from build123d import *

# Parameters (mm, degrees)
BOSS_EXTRUDE1_DEPTH   = 38.1
BOSS_EXTRUDE1_2_DEPTH = 38.1
SKETCH2_W             = 7.62
SKETCH2_H             = 5.08
BOSS_EXTRUDE2_DEPTH   = 7.62
SKETCH3_R             = 1.8415
CUT_EXTRUDE1_DEPTH    = 60.428216724
FILLET1_R             = 2.54
FILLET2_R             = 2.54
SKETCH5_W             = 18.161
SKETCH5_H             = 5.08
SKETCH5_W_2           = 21.209
BOSS_EXTRUDE3_DEPTH   = 5.08
SKETCH6_W             = 8.89
SKETCH6_H             = 27.94
CUT_EXTRUDE2_DEPTH    = 63.393930338
SKETCH8_W             = 8.763
SKETCH8_H             = 3.302
BOSS_EXTRUDE4_DEPTH   = 13.97
SKETCH11_R            = 1.8415
CUT_EXTRUDE4_DEPTH    = 62.324385256
CUT_EXTRUDE5_START    = -5.08
SKETCH15_W            = 35.43046
SKETCH15_H            = 22.86
CUT_EXTRUDE5_DEPTH    = 5.08
SKETCH16_R            = 1.8415
BOSS_EXTRUDE5_DEPTH   = 5.08
SKETCH17_W            = 5.08
SKETCH17_H            = 21.717
CUT_EXTRUDE6_DEPTH    = 10.16
CHAMFER1_SIZE         = 2.54


with BuildPart() as part:
    # Sketch1 → Boss-Extrude1 (new body)
    with BuildSketch(Plane(origin=(0, 0, 0), x_dir=(1, 0, 0), z_dir=(0, 1, 0))):
        Polygon((0, 0), (0, 13.71346), (5.08, 13.71346), (5.08, 5.588), (19.05, 5.588), (19.05, 0), align=None)
    extrude(amount=BOSS_EXTRUDE1_DEPTH)

    # Sketch2 → Boss-Extrude2 (add)
    with BuildSketch(Plane.ZY):
        with Locations((-6.85546, 35.56)):
            Rectangle(SKETCH2_W, SKETCH2_H)
        with Locations((-38.73246, 35.56)):
            Rectangle(SKETCH2_W, SKETCH2_H)
    extrude(amount=BOSS_EXTRUDE2_DEPTH)


with BuildPart() as body_2:
    # Sketch1 → Boss-Extrude1 2 (new body)
    with BuildSketch(Plane(origin=(0, 0, 0), x_dir=(1, 0, 0), z_dir=(0, 1, 0))):
        Polygon((0, 31.87446), (5.08, 31.87446), (5.08, 40.00246), (19.05, 40.00246), (19.05, 45.59046), (0, 45.59046), align=None)
    extrude(amount=BOSS_EXTRUDE1_2_DEPTH)



with BuildPart() as boss_extrude2_piece_1:
    # of the separate pieces the step leaves, piece 1, a body of its own (boss_extrude2_pieces)
    add(part.part.solids().sort_by_distance((0, 0, 0))[0])


with BuildPart() as boss_extrude2_piece_2:
    # of the separate pieces the step leaves, piece 2, a body of its own (boss_extrude2_pieces)
    add(part.part.solids().sort_by_distance((0, 38.1, -34.92246))[0])


with BuildPart() as cut_extrude1_tool:
    # Sketch3 → Cut-Extrude1 (new, through all)
    with BuildSketch(Plane(origin=(0, 33.02, 0), x_dir=(-1, 0, 0), z_dir=(0, -1, 0))):
        with Locations(Location((3.996511692, 6.85546, 0), (0, 0, 90))):
            Circle(SKETCH3_R)
        with Locations(Location((3.996511692, 38.73246, 0), (0, 0, 90))):
            Circle(SKETCH3_R)
    extrude(amount=-CUT_EXTRUDE1_DEPTH)


with BuildPart() as boss_extrude2_piece_1_1:
    add(boss_extrude2_piece_1.part)

    # Cut-Extrude1: cut by cut_extrude1_tool
    add(cut_extrude1_tool.part, mode=Mode.SUBTRACT)

    # Fillet1
    fillet1_edges = [boss_extrude2_piece_1_1.edges().sort_by_distance(p)[0] for p in [
        (-7.62, 35.56, -10.66546),
        (-7.62, 35.56, -3.04546),
    ]]
    fillet(fillet1_edges, radius=FILLET1_R)


with BuildPart() as boss_extrude2_piece_2_1:
    add(boss_extrude2_piece_2.part)

    # Cut-Extrude1: cut by cut_extrude1_tool
    add(cut_extrude1_tool.part, mode=Mode.SUBTRACT)

    # Fillet2
    fillet2_edges = [boss_extrude2_piece_2_1.edges().sort_by_distance(p)[0] for p in [
        (-7.62, 35.56, -42.54246),
        (-7.62, 35.56, -34.92246),
    ]]
    fillet(fillet2_edges, radius=FILLET2_R)


with BuildPart() as body_2_1:
    add(body_2.part)

    add(boss_extrude2_piece_1_1.part)  # Boss-Extrude3 merges Boss-Extrude2 piece 1

    add(boss_extrude2_piece_2_1.part)  # Boss-Extrude3 merges Boss-Extrude2 piece 2
    # Sketch5 → Boss-Extrude3 (add)
    with BuildSketch(Plane.ZY):
        with Locations((-22.79396, 2.54)):
            Rectangle(SKETCH5_W, SKETCH5_H)
        with Locations((-24.31796, 30.48)):
            Rectangle(SKETCH5_W_2, SKETCH5_H)
    extrude(amount=-BOSS_EXTRUDE3_DEPTH)

    # Sketch6 → Cut-Extrude2 (cut, through all)
    with BuildSketch(Plane.XY):
        with Locations((9.525, 19.05)):
            Rectangle(SKETCH6_W, SKETCH6_H)
    extrude(amount=-CUT_EXTRUDE2_DEPTH, mode=Mode.SUBTRACT)

    # Sketch8 → Boss-Extrude4 (add)
    with BuildSketch(Plane(origin=(5.08, 0, 0), x_dir=(0, 0, -1), z_dir=(1, 0, 0))):
        with Locations((9.9695, 3.429)):
            Rectangle(SKETCH8_W, SKETCH8_H)
        with Locations((35.62096, 3.429)):
            Rectangle(SKETCH8_W, SKETCH8_H)
    extrude(amount=BOSS_EXTRUDE4_DEPTH)

    # Sketch11 → Cut-Extrude4 (cut, through all)
    with BuildSketch(Plane.XZ.offset(-1.778)):
        with Locations(Location((13.1064, -9.7028, 0), (0, 0, 270))):
            Circle(SKETCH11_R)
        with Locations(Location((13.1064, -35.88766, 0), (0, 0, 270))):
            Circle(SKETCH11_R)
    extrude(amount=-CUT_EXTRUDE4_DEPTH, mode=Mode.SUBTRACT)

    # Sketch15 → Cut-Extrude5 (cut)
    with BuildSketch(Plane.ZY.offset(CUT_EXTRUDE5_START)):
        with Locations((-22.79523, 16.51)):
            Rectangle(SKETCH15_W, SKETCH15_H)
    extrude(amount=CUT_EXTRUDE5_DEPTH, mode=Mode.SUBTRACT)

    # Sketch16 → Boss-Extrude5 (add)
    # profile 1 of 2: a face of its own
    with BuildSketch(Plane(origin=(0, 38.1, 0), x_dir=(1, 0, 0), z_dir=(0, 1, 0))):
        with BuildLine():
            Line((-3.996511692, 43.81246), (3.107709624, 43.81246))
            Line((3.107709624, 43.81246), (3.042520574, 33.65246))
            Line((3.042520574, 33.65246), (-3.996511692, 33.65246))
            ThreePointArc((-3.996511692, 33.65246), (-9.076511692, 38.73246), (-3.996511692, 43.81246))
        make_face()
        with Locations(Location((-3.996511692, 38.73246, 0), (0, 0, 90))):
            Circle(SKETCH16_R, mode=Mode.SUBTRACT)
    # profile 2 of 2: a face of its own
    with BuildSketch(Plane(origin=(0, 38.1, 0), x_dir=(1, 0, 0), z_dir=(0, 1, 0))):
        with BuildLine():
            Line((-3.996511692, 11.93546), (2.83798993, 11.93546))
            ThreePointArc((2.83798993, 11.93546), (2.870583784, 11.935355436), (2.903176296, 11.935041748))
            Line((2.903176296, 11.935041748), (2.83798993, 1.77546))
            Line((2.83798993, 1.77546), (-3.996511692, 1.77546))
            ThreePointArc((-3.996511692, 1.77546), (-9.076511692, 6.85546), (-3.996511692, 11.93546))
        make_face()
        with Locations(Location((-3.996511692, 6.85546, 0), (0, 0, 90))):
            Circle(SKETCH16_R, mode=Mode.SUBTRACT)
    extrude(amount=-BOSS_EXTRUDE5_DEPTH)

    # Sketch17 → Cut-Extrude6 (cut)
    with BuildSketch(Plane(origin=(0, 38.1, 0), x_dir=(1, 0, 0), z_dir=(0, 1, 0))):
        with Locations((2.54, 22.79396)):
            Rectangle(SKETCH17_W, SKETCH17_H)
    extrude(amount=-CUT_EXTRUDE6_DEPTH, mode=Mode.SUBTRACT)

    # Chamfer1
    chamfer1_edges = [body_2_1.edges().sort_by_distance(p)[0] for p in [
        (5.08, 35.56, -40.00246),
        (5.08, 35.56, -5.588),
    ]]
    chamfer(chamfer1_edges, length=CHAMFER1_SIZE)


solid = body_2_1.part
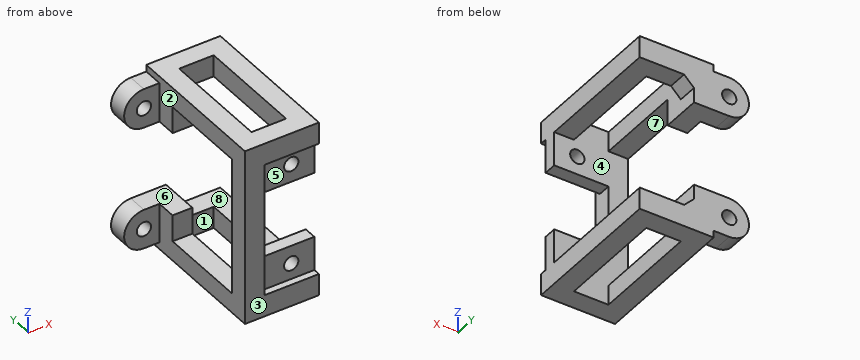
Could you check a few things on this model? Use its own coordinates, in mm. Face numbers are marked on the shaded views. A direction names the side the tool comes from. Give positions to 0.01 mm unless a question says otherwise; leave off trailing zeros. Order: outer loops, then holes, each group sorted by start corner. A loop starts at its lowest first (then second) coordinate and runs counter-clockwise, first axis right, second up.
Item 1: If we section it at B-B, the plane x = 16.75: Write out the boundary of the cut face in (y, z), plus the area to 3 significant figures.
Item 2: I need wall thicknesses on line 1 (Y direction, x = 1.25, z = -10.5); line 2 (Y direction, x = -0.25, z = -40); line 3 (X direction, y = 3, z = -22.5). Which ranges of each line are inside material? Lowest first, please.
Item 3: If we section it at D-D, the plane z = -39: Write out the boundary of the cut face in (x, y).
Item 4: If we section it at A-A, the plane y = 26: Write out the boundary of the cut face in (x, z).
Item 5: I'm going to push flat-ended pins straight in: pin 1 (2.5 mm diameter, centred on x = -6, z = -37.5, fed in from -Y); pin 2 (12 mm diameter, centred on y = 10.5, z = -28, fed in from -X); pin 3 (6 mm diameter, centred on x = -2, z = -26, fed in from +Y); pin 4 (10 mm diameter, centred on x = 14.5, z = -23.5, fed in from -Y). Where does each tip first touch, or does it pass through?
Item 6: If we section it at C-C, the plane x = 10.5: Write out the boundary of the cut face in (y, z).
Item 7: If we mould it in two halves opening along Y, with no side actions, what happens to the marked faces 1, 2, 3 and 4? For each: pulls with the +Y half, pulls with the -Y half, needs draft (parallel to the pull), parting line crosses it, or undercut.
Item 8: For the marked faces 5, 6, 7 and 8, which set-ups out of +Z, -Z, +X, -X, +Y, -Y let a thin tool reach every point of the face, with its end or its side?
Values:
1. outline: (0, -45.59) - (38.1, -45.59) - (38.1, -40) - (5.08, -40) - (5.08, -31.24) - (1.78, -31.24) - (1.78, -40) - (0, -40) - close; (0, -5.59) - (1.78, -5.59) - (1.78, -14.35) - (5.08, -14.35) - (5.08, -5.59) - (38.1, -5.59) - (38.1, 0) - (0, 0) - close
1. area: 484 mm2
2. line 1: y = 0 to 5.08, 27.94 to 38.1
2. line 2: y = 33.02 to 38.1
2. line 3: x = 0 to 5.08
3. outline: (-9.07, 33.02) - (-5.82, 33.02) - (-5.82, 38.1) - (-9.07, 38.1) - close; (-2.17, 33.02) - (0, 33.02) - (0, 27.94) - (5.08, 27.94) - (5.08, 33.02) - (6.62, 33.02) - (6.62, 38.1) - (-2.17, 38.1) - close; (0, 0) - (5.08, 0) - (5.08, 1.78) - (19.05, 1.78) - (19.05, 5.08) - (0, 5.08) - close
4. outline: (0, -45.59) - (5.08, -45.59) - (5.08, -40.51) - (0, -40.51) - close; (0, -5.08) - (5.08, -5.08) - (5.08, 0) - (0, 0) - close; (13.97, -45.59) - (19.05, -45.59) - (19.05, -40) - (13.97, -40) - close; (13.97, -5.59) - (19.05, -5.59) - (19.05, 0) - (13.97, 0) - close
5. pin 1: stops at y = 33.02
5. pin 2: stops at x = 0
5. pin 3: stops at y = 5.08
5. pin 4: passes through
6. outline: (0, -45.59) - (5.08, -45.59) - (5.08, -31.24) - (1.78, -31.24) - (1.78, -40) - (0, -40) - close; (0, -5.59) - (1.78, -5.59) - (1.78, -14.35) - (5.08, -14.35) - (5.08, 0) - (0, 0) - close; (33.02, -45.59) - (38.1, -45.59) - (38.1, -40) - (33.02, -40) - close; (33.02, -5.59) - (38.1, -5.59) - (38.1, 0) - (33.02, 0) - close
7. face 1: undercut
7. face 2: needs draft
7. face 3: pulls with the -Y half
7. face 4: undercut
8. face 5: +X, -Y
8. face 6: +X, -X, +Y
8. face 7: -X
8. face 8: +X, +Y
